from build123d import *

# Parameters (mm, degrees)
SKETCH1_R               = 6
BOSS_EXTRUDE1_DEPTH     = 260
CHAMFER1_SIZE           = 1
SKETCH3_W               = 3
SKETCH3_H               = 30
SKETCH3_W_2             = 2
SKETCH3_H_2             = 10
SKETCH3_H_3             = 5
CUT_EXTRUDE1_DEPTH      = 7
CUT_EXTRUDE1_DEPTH_BACK = 7
SKETCH4_R               = 3
CUT_EXTRUDE2_DEPTH      = 3
CUT_EXTRUDE2_DEPTH_BACK = 11
SKETCH5_W               = 10
SKETCH5_H               = 1.527864045
SKETCH5_W_2             = 5
CUT_EXTRUDE3_DEPTH      = 7
CUT_EXTRUDE3_DEPTH_BACK = 7


with BuildPart() as part:
    # Sketch1 → Boss-Extrude1 (new body)
    with BuildSketch(Plane.XY):
        Circle(SKETCH1_R)
    extrude(amount=BOSS_EXTRUDE1_DEPTH)

    # Chamfer1
    chamfer1_edges = [part.edges().sort_by_distance(p)[0] for p in [
        (-6, 0, 0),
        (-6, 0, 260),
    ]]
    chamfer(chamfer1_edges, length=CHAMFER1_SIZE)

    # Sketch3 → Cut-Extrude1 (cut, two sides)
    with BuildSketch(Plane(origin=(0, 0, 0), x_dir=(1, 0, 0), z_dir=(0, 1, 0))) as cut_extrude1_sk:
        with Locations((4.5, -245)):
            Rectangle(SKETCH3_W, SKETCH3_H)
        with Locations((5, -154.5)):
            Rectangle(SKETCH3_W_2, SKETCH3_H_2)
        with Locations((-5, -154.5)):
            Rectangle(SKETCH3_W_2, SKETCH3_H_2)
        with Locations((5, -121.5)):
            Rectangle(SKETCH3_W_2, SKETCH3_H_3)
    extrude(amount=CUT_EXTRUDE1_DEPTH, mode=Mode.SUBTRACT)
    extrude(cut_extrude1_sk.sketch, amount=-CUT_EXTRUDE1_DEPTH_BACK, mode=Mode.SUBTRACT)

    # Sketch4 → Cut-Extrude2 (cut, two sides)
    with BuildSketch(Plane(origin=(4, 0, 0), x_dir=(0, 0, -1), z_dir=(1, 0, 0))) as cut_extrude2_sk:
        with Locations((-154.5, 0)):
            Circle(SKETCH4_R)
    extrude(amount=CUT_EXTRUDE2_DEPTH, mode=Mode.SUBTRACT)
    extrude(cut_extrude2_sk.sketch, amount=-CUT_EXTRUDE2_DEPTH_BACK, mode=Mode.SUBTRACT)

    # Sketch5 → Cut-Extrude3 (cut, two sides)
    with BuildSketch(Plane(origin=(0, 0, 0), x_dir=(0, 0, -1), z_dir=(1, 0, 0))) as cut_extrude3_sk:
        with Locations((-154.5, 5.236067978)):
            Rectangle(SKETCH5_W, SKETCH5_H)
        with Locations((-121.5, 5.236067978)):
            Rectangle(SKETCH5_W_2, SKETCH5_H)
    extrude(amount=CUT_EXTRUDE3_DEPTH, mode=Mode.SUBTRACT)
    extrude(cut_extrude3_sk.sketch, amount=-CUT_EXTRUDE3_DEPTH_BACK, mode=Mode.SUBTRACT)


solid = part.part
Verification items for the finished model (mm, model axes). A direction names the side the tool comes from. Give positions to 0.01 mm unless a question says otherwise; leave off trailing zeros. Loops run counter-clockwise (first coordinate to the right, second up) from the corner with the lowest first, then second, coordinate; pieces in that order, holes last. Notation, with made-up numbers: (51, 47.25) - (102, 47.25) arc R9 cw to (102, 54.25) - close; hole circle Ø2 at (3.5, 44.25). An arc over 180 degrees is marked (long way). Write each question's results on one line, items separated by ' | '.
1) Tool access check on faces 4 (the flat face through (-4, 2, 157)), 5 (the flat face through (3, 0, 245)), 6 (the cylindrical face through (-4.76, -3.65, 128.19)), 7 (the flat face through (4, 2, 157)), 8 (the flat face through (0, 4.472, 155)). Record the directions out of +Z, -Z, +X, -X, +Y, -Y that give a thin tool (end or side, any length) a straight path to the whole face; none if there is none.
Solution:
face 4: -X, +Y, -Y | face 5: +Z, +X, +Y, -Y | face 6: +Z, -Z | face 7: +X, +Y, -Y | face 8: +X, -X, +Y
2) Depth check by flat-ended pin: P1, Ø1, axis at x = 5.5, y = -1.5, coming from the +Z side; P2, Ø2.5, axis at y = -1, z = 122, coming from the +X side; P3, Ø0.5, axis at x = 0.5, y = 5.5, coming from the -Z side; P4, Ø5.5, axis at y = 0, z = 154.5, coming from the +X side. Enter the tip coordinate at first touch or a pass-through.
Solution:
P1: z = 230 | P2: x = 4 | P3: z = 0.27 | P4: through
3) Material ranges on L1, parallel to Y at x = 0.25, z = 154.5; L2, parallel to Y at x = -0.5, z = 43.5; L3, parallel to Y at x = 3.25, z = 160, recorded low to high. Write a range as from..to.
Solution:
L1: -5.99..-3, 3..4.47 | L2: -5.98..5.98 | L3: -5.04..5.04
4) Mould release check, pull along Z, two halves, no side actions. Record for faces 1 (the flat face through (0, 0, 0)), 2 (the conical face through (-5.16, 0.16, 259.84)), 3 (the flat face through (4, 0, 122)): pulls with the +Z half, pulls with the -Z half, needs draft (parallel to the pull), parting line crosses it, or undercut.
Solution:
face 1: pulls with the -Z half | face 2: pulls with the +Z half | face 3: undercut
5) Sectioned sample at D-D on z = 63. Record the boundary of the cut face in (x, y).
Solution:
outline: circle Ø12 at (0, 0)
6) Sectioned sample at A-A on z = 154.5. Record the boundary of the cut face in (x, y).
Solution:
outline: (-4, -4.47) arc R6 ccw to (4, -4.47) - (4, -3) - (-4, -3) - close; (-4, 3) - (4, 3) - (4, 4.47) - (-4, 4.47) - close
7) Sectioned sample at B-B on x = 0. Record the boundary of the cut face in (y, z), plus the area to 3 significant figures.
Solution:
outline: (-6, 1) - (-5, 0) - (5, 0) - (6, 1) - (6, 119) - (4.47, 119) - (4.47, 124) - (6, 124) - (6, 149.5) - (4.47, 149.5) - (4.47, 159.5) - (6, 159.5) - (6, 259) - (5, 260) - (-5, 260) - (-6, 259) - close; hole circle Ø6 at (0, 154.5) | area: 3,070 mm2
8) Sectioned sample at C-C on y = 0. Record the boundary of the cut face in (x, z), plus the area to 3 significant figures.
Solution:
outline: (-6, 1) - (-5, 0) - (5, 0) - (6, 1) - (6, 119) - (4, 119) - (4, 124) - (6, 124) - (6, 149.5) - (4, 149.5) - (4, 151.5) - (-4, 151.5) - (-4, 149.5) - (-6, 149.5) - close; (-6, 159.5) - (-4, 159.5) - (-4, 157.5) - (4, 157.5) - (4, 159.5) - (6, 159.5) - (6, 230) - (3, 230) - (3, 260) - (-5, 260) - (-6, 259) - close | area: 2,930 mm2
